Design review of the part built by this model. Coordinates are the model's own, in mm. A direction names the side the tool comes from. Coordinates: 2 decimals unless noted, no trailing zeros. Order: outer loops, then holes, each group sorted by start corner. A loop starts at its lowest first (then second) coordinate and runs counter-clockwise, first axis right, second up. Notation, with made-up numbers: (43.25, 88) -> (94.25, 88) arc R29 ccw to (94.25, 113) -> close; hole circle Ø5 at (74, 71.5). An arc over 180 degrees is marked (long way). Write item = value, one per line.
```python
from build123d import *

# Parameters (mm, degrees)
BOSS_EXTRUDE1_DEPTH                                 = 10.568712475
CBORE_FOR_4_BINDING_HEAD_MACHINE_SCREW1_D           = 3.2639
CBORE_FOR_4_BINDING_HEAD_MACHINE_SCREW1_CBORE_D     = 6.74624
CBORE_FOR_4_BINDING_HEAD_MACHINE_SCREW1_CBORE_DEPTH = 1.7272
CBORE_FOR_4_BINDING_HEAD_MACHINE_SCREW2_D           = 3.2639
CBORE_FOR_4_BINDING_HEAD_MACHINE_SCREW2_CBORE_D     = 6.74624
CBORE_FOR_4_BINDING_HEAD_MACHINE_SCREW2_CBORE_DEPTH = 1.7272


with BuildPart() as part:
    # Sketch1 → Boss-Extrude1 (new body)
    with BuildSketch(Plane.XY):
        with BuildLine():
            Line((0, -9.926359007), (-108.863033935, -9.926359007))
            ThreePointArc((-108.863033935, -9.926359007), (-118.789392942, 0), (-108.863033935, 9.926359007))
            Line((-108.863033935, 9.926359007), (0, 9.926359007))
            ThreePointArc((0, 9.926359007), (9.926359007, 0), (0, -9.926359007))
        make_face()
    extrude(amount=BOSS_EXTRUDE1_DEPTH)

    # CBORE for #4 Binding Head Machine Screw1 (through all)
    with Locations(Plane.XY.offset(10.568712475)):
        with Locations((-2.744321225, 0)):
            CounterBoreHole(CBORE_FOR_4_BINDING_HEAD_MACHINE_SCREW1_D / 2, CBORE_FOR_4_BINDING_HEAD_MACHINE_SCREW1_CBORE_D / 2, CBORE_FOR_4_BINDING_HEAD_MACHINE_SCREW1_CBORE_DEPTH)

    # CBORE for #4 Binding Head Machine Screw2 (through all)
    with Locations(Plane.XY.offset(10.568712475)):
        with Locations((-108.687959282, 0)):
            CounterBoreHole(CBORE_FOR_4_BINDING_HEAD_MACHINE_SCREW2_D / 2, CBORE_FOR_4_BINDING_HEAD_MACHINE_SCREW2_CBORE_D / 2, CBORE_FOR_4_BINDING_HEAD_MACHINE_SCREW2_CBORE_DEPTH)


solid = part.part
```
(1) We need section A-A (y = 0). Write out the cut boundary in (x, z).
Report:
outline = (-118.79, 0) -> (-110.32, 0) -> (-110.32, 8.84) -> (-112.06, 8.84) -> (-112.06, 10.57) -> (-118.79, 10.57) -> close; (-107.06, 0) -> (-4.38, 0) -> (-4.38, 8.84) -> (-6.12, 8.84) -> (-6.12, 10.57) -> (-105.31, 10.57) -> (-105.31, 8.84) -> (-107.06, 8.84) -> close; (-1.11, 0) -> (9.93, 0) -> (9.93, 10.57) -> (0.63, 10.57) -> (0.63, 8.84) -> (-1.11, 8.84) -> close
(2) Insertion check: pin 1 (3 mm diameter, centred on x = -2.74, y = 0, fed in from +Z); pin 2 (4 mm diameter, centred on y = 3, z = 8.5, fed in from -X); pin 3 (1.5 mm diameter, centred on y = -1, z = 2.5, fed in from +X); pin 4 (4 mm diameter, centred on y = 5.5, z = 6.5, fed in from -X). Each pin has a flat end and moves straight along its axis. Give the tip position at first contact, or say it passes through.
Report:
pin_1 = through
pin_2 = -118.74
pin_3 = 9.92
pin_4 = -118.15
(3) The part is to be moulded in two halves that separate along Y. For faces 1 (the flat face through (-54, -9.926, 5)), 2 (the cylindrical face through (-107.058, 0.072, 4.359)), 3 (the flat face through (-55, 9.926, 5)), 4 (the cylindrical face through (9.924, 0.218, 5.21)), say which applies: released by +Y, released by -Y, zero draft, split by the parting line, or undercut.
Report:
face_1 = released by -Y
face_2 = undercut
face_3 = released by +Y
face_4 = split by the parting line
(4) We need section D-D (y = 8.75). Write out the cut boundary in (x, z), and give its area (3 significant figures).
Report:
outline = (-113.55, 0) -> (4.69, 0) -> (4.69, 10.57) -> (-113.55, 10.57) -> close
area = 1,250 mm²
(5) For faces 5 (the flat face through (-54, 0, 0)), 6 (the flat face through (-107, 1, 8.842)), list the 3-axis set-ups (+Z, -Z, +X, -X, +Y, -Y) from which the entire face can be reached by the end or side of a thin tool; tool diameter is ignored.
Report:
face_5 = -Z, +X, -X, +Y, -Y
face_6 = +Z
(6) We need section B-B (z = 1.75). Write out the cut boundary in (x, y), and give its area (3 significant figures).
Report:
outline = (-108.86, -9.93) -> (0, -9.93) arc R9.93 ccw to (0, 9.93) -> (-108.86, 9.93) arc R9.93 ccw to start; hole circle Ø3.26 at (-108.69, 0); hole circle Ø3.26 at (-2.74, 0)
area = 2,450 mm²
(7) For L1, parallel to X at y = -1, z = 3.75; L2, parallel to Y at x = -3, z = 10; L3, parallel to X at y = -2.25, z = 10, list the stretches that pass through material, from the lowest coordinate up.
Report:
L1 = -118.74 to -109.98, -107.4 to -4.03, -1.45 to 9.88
L2 = -9.93 to -3.36, 3.36 to 9.93
L3 = -118.53 to -111.2, -106.17 to -5.26, -0.23 to 9.67
(8) We need section C-C (y = -6.75). Write out the cut boundary in (x, z), and give its area (3 significant figures).
Report:
outline = (-116.14, 0) -> (7.28, 0) -> (7.28, 10.57) -> (-116.14, 10.57) -> close
area = 1,300 mm²
